Input: part model. Units: mm. Frame: model coordinates. A direction names the side the tool comes from. Give positions to 0.01 mm unless a question says otherwise; leave off trailing zeros. Answer as a JSON object with one key per item and string values.
```python
from build123d import *

# Parameters (mm, degrees)
BOSS_EXTRU_1_DEPTH           = 729
ENL_V_MAT_EXTRU_1_DEPTH      = 727
ESQUISSE3_W                  = 40
ESQUISSE3_H                  = 40
BOSS_EXTRU_2_DEPTH           = 814.58026
ENL_V_MAT_EXTRU_2_DEPTH      = 829.69546376
ENL_V_MAT_EXTRU_2_DEPTH_BACK = 829.69546376
ESQUISSE4_W                  = 98.578400591
ESQUISSE4_H                  = 147.950096535
ESQUISSE4_W_2                = 77.840885054
ESQUISSE4_H_2                = 46.084081252
ESQUISSE7_W                  = 821.544509843
ESQUISSE7_H                  = 616.158382383
ESQUISSE7_W_2                = 40
ESQUISSE7_H_2                = 40
ENL_V_MAT_EXTRU_6_DEPTH      = 828.213294061
ESQUISSE8_W                  = 32
ESQUISSE8_H                  = 32
ENL_V_MAT_EXTRU_9_DEPTH      = 828.213294061
CONG_2_R                     = 2


with BuildPart() as part:
    # Esquisse1 → Boss.-Extru.1 (new body)
    with BuildSketch(Plane.XY):
        Polygon((0, 0), (258, 0), (0, 256), align=None)
    extrude(amount=BOSS_EXTRU_1_DEPTH)

    # Esquisse2 → Enlèv. mat.-Extru.1 (cut)
    with BuildSketch(Plane.ZY):
        Polygon((0, 256), (729, 0), (729, 256), align=None)
    extrude(amount=-ENL_V_MAT_EXTRU_1_DEPTH, mode=Mode.SUBTRACT)

    # Esquisse3 → Boss.-Extru.2 (add)
    with BuildSketch(Plane(origin=(0, 256, 0), x_dir=(0.948516525956314, 0.10519863837129277, -0.2987467932423567), z_dir=(0.31672753768478995, -0.31427228545467534, 0.8949394378767902))):
        with Locations((20, -20)):
            Rectangle(ESQUISSE3_W, ESQUISSE3_H)
    extrude(amount=BOSS_EXTRU_2_DEPTH)

    # Esquisse4 → Enlèv. mat.-Extru.2 (cut, two sides: drawn at the far end of the back side and taken through both)
    with BuildSketch(Plane(origin=(0, 0, 0), x_dir=(-1, 0, 0), z_dir=(0, -1, 0)).offset(-ENL_V_MAT_EXTRU_2_DEPTH_BACK)):
        with Locations((-307.289200295, -655.024951733)):
            Rectangle(ESQUISSE4_W, ESQUISSE4_H)
        with Locations((-38.920442527, 23.042040626)):
            Rectangle(ESQUISSE4_W_2, ESQUISSE4_H_2)
    extrude(amount=ENL_V_MAT_EXTRU_2_DEPTH + ENL_V_MAT_EXTRU_2_DEPTH_BACK, mode=Mode.SUBTRACT)

    # Esquisse7 → Enlèv. mat.-Extru.6 (cut, through all)
    with BuildSketch(Plane(origin=(0, 256, 0), x_dir=(0.948516525956314, 0.10519863837129277, -0.2987467932423567), z_dir=(0.31672753768478995, -0.31427228545467534, 0.8949394378767902))):
        with Locations((22.907114777, -53.97111912)):
            Rectangle(ESQUISSE7_W, ESQUISSE7_H)
        with Locations((20, -20)):
            Rectangle(ESQUISSE7_W_2, ESQUISSE7_H_2, mode=Mode.SUBTRACT)
    extrude(amount=ENL_V_MAT_EXTRU_6_DEPTH, mode=Mode.SUBTRACT)

    # Esquisse8 → Enlèv. mat.-Extru.9 (cut, through all)
    with BuildSketch(Plane(origin=(0, 256, 0), x_dir=(0.948516525956314, 0.10519863837129277, -0.2987467932423567), z_dir=(0.31672753768478995, -0.31427228545467534, 0.8949394378767902))):
        with Locations((20, -20)):
            Rectangle(ESQUISSE8_W, ESQUISSE8_H)
    extrude(amount=ENL_V_MAT_EXTRU_9_DEPTH, mode=Mode.SUBTRACT)

    # Congé2
    cong_2_edges = [part.edges().sort_by_distance(p)[0] for p in [
        (131.343588352, 126.087109834, 357.878000354),
        (133.224361668, 94.037568496, 352.563722265),
        (150.092295167, 110.783988508, 304.90200319),
        (148.211521852, 142.833529846, 310.21628128),
        (129, 128, 364.5),
        (150.084916875, 148.933025015, 304.922851157),
        (152.435883519, 108.871098342, 298.280003544),
        (131.350966645, 87.938073327, 357.857152388),
    ]]
    fillet(cong_2_edges, radius=CONG_2_R)


solid = part.part
```
Q1. Pin query (flat end, axial travel): pin 1 (3 mm diameter, centred on y = 104.5, z = 393.5, fed in from +X). Return the tip coordinate at first contact, or that it passes through.
Evaluation:
{"pin 1": "stops at x = 183.41"}
Q2. Draft query along Z for faces 1 (the flat face through (129.693, 112.448, 347.835)), 2 (the cylindrical face through (130, 90.44, 352.54)), 3 (the cylindrical face through (131.4, 125.65, 369.38)), 4 (the cylindrical face through (151.88, 108.92, 311.93)). Return one class per face: +Z half, -Z half, draft (parallel to the pull), parting line (faces both ways), or undercut.
Evaluation:
{"face 1": "undercut", "face 2": "parting line", "face 3": "+Z half", "face 4": "undercut"}
Q3. Access query for faces 5 (the flat face through (258, -12, 653)), 6 (the cylindrical face through (135.397, 93.046, 357.203)). Directions: +Z, -Z, +X, -X, +Y, -Y. A direction counts if a zero-diameter tool reaches every point of the face in a straight line with its end or side. Return the directions, or none.
Evaluation:
{"face 5": "+Z, -Z, +X, +Y, -Y", "face 6": "none"}
Q4. Ray query, line 1 along X through (y, z) = (105, 361.5); line 2 along Y through (x, z) = (42, 85.5); line 3 along Y through (x, z) = (76, 160). Return the intervals inside material, ascending.
Evaluation:
{"line 1": "x = 130.61 to 134.82, 168.56 to 172.78", "line 2": "y = 183.58 to 187.82, 221.74 to 225.98", "line 3": "y = 157.42 to 161.66, 195.58 to 199.82"}
